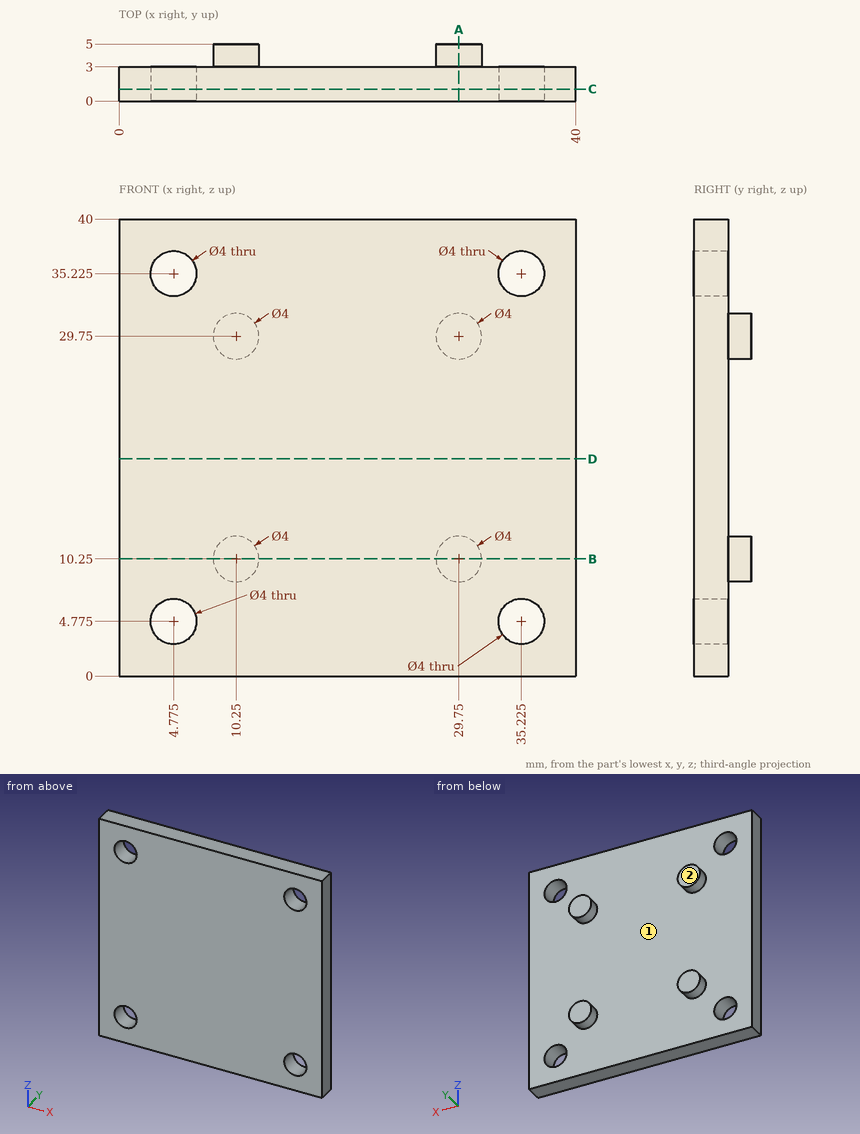
Input: dimensioned drawing with shaded views. Units: mm. Origin: part minimum x, y, z. A direction names the side the tool comes from. Give positions to 0.01 mm unless a question says otherwise; leave off trailing zeros. Loops run counter-clockwise (first coordinate to the right, second up) from the corner with the lowest first, then second, coordinate; pieces in that order, holes last. Notation, with made-up numbers: M -29.75,-22 L -12.75,-22 A29 ccw -12.75,6 Z; hole C -8,54.25 d4. An arc over 180 degrees is marked long. Put each result on its own line as item: value. Start each with the question number.
1) Cut plane B-B (z = 10.25). Output: boundary loops of the cut face in (x, y).
2) Contact query for a flat-ended pin moving along its axis: pin 1 (5 mm diameter, centred on x = 4.78, z = 4.78, fed in from +Y). Output: stop coordinate, or through.
3) Access query for the marked faces 1 and 2. Directions: +Z, -Z, +X, -X, +Y, -Y. A direction counts if a zero-diameter tool reaches every point of the face in a straight line with its end or side. Return the directions, or none.
4) Ray query, line 1 along Z through (x, y) = (5, 2.4); line 2 along Z through (x, y) = (6.5, 2.25); line 3 along Y through (x, z) = (17.5, 6.5). Return the intervals inside material, ascending.
5) Cut plane C-C (y = 1.05). Output: boundary loops of the cut face in (x, z) (1 decimal).
6) Cut plane D-D (z = 19). Output: boundary loops of the cut face in (x, y), then the cut area to 3 significant figures.
7) Cut plane A-A (x = 29.75). Output: boundary loops of the cut face in (y, z).
Verdict:
1. outline: M 0,0 L 40,0 L 40,3 L 31.75,3 L 31.75,5 L 27.75,5 L 27.75,3 L 12.25,3 L 12.25,5 L 8.25,5 L 8.25,3 L 0,3 Z
2. pin 1: y = 3
3. face 1: +Y
3. face 2: +Z, -Z, +X, -X, +Y
4. line 1: 0 to 2.79, 6.76 to 33.24, 37.21 to 40
4. line 2: 0 to 3.76, 5.79 to 34.21, 36.24 to 40
4. line 3: 0 to 3
5. outline: M 0,0 L 40,0 L 40,40 L 0,40 Z; hole C 4.8,4.8 d4; hole C 4.8,35.2 d4; hole C 35.2,4.8 d4; hole C 35.2,35.2 d4
6. outline: M 0,0 L 40,0 L 40,3 L 0,3 Z
6. area: 120 mm2
7. outline: M 0,0 L 3,0 L 3,8.25 L 5,8.25 L 5,12.25 L 3,12.25 L 3,27.75 L 5,27.75 L 5,31.75 L 3,31.75 L 3,40 L 0,40 Z
